Can you work these out from the model? Positions are in its coordinate system, mm. Face numbers are marked on the shaded views. A direction names the side the tool comes from. Round coordinates to 2 decimals unless told otherwise and drop trailing zeros. Loops run counter-clockwise (first coordinate to the right, second up) from the corner with the lowest first, then second, coordinate; pieces in that order, holes last.
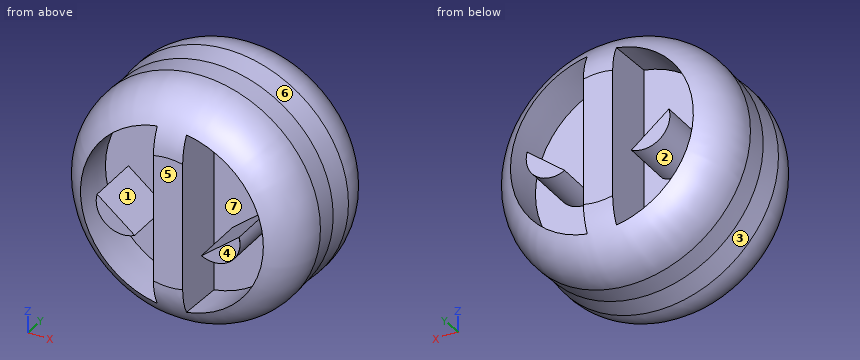
from build123d import *

# Parameters (mm, degrees)
F0_R         = 55.5262746105
F1_DEPTH     = 38.1
F1_TAPER     = -3
F2_DEPTH     = 38.1
F3_DEPTH     = 12.7
F4_DEPTH     = 38.1
F5_S5_R      = 12.3526687507
F5_T6_DEPTH  = 90
F5_S7_R      = 12.3526687507
F5_T8_DEPTH  = 90
F5_S13_R     = 12.3526687507
F5_T14_DEPTH = 90
F5_S15_R     = 12.3526687507
F5_T16_DEPTH = 90


# Not quite as in the source:
# - a fillet or chamfer that OpenCascade refuses, or shapes differently, is made with other operations: its cross-section is extruded or revolved along the edge and cut away or added
# - two fillets or chamfers of one size are made in one step


with BuildPart() as f1:
    # F0 (on Front) → F1 (new body, symmetric)
    with BuildSketch(Plane.XZ):
        Circle(F0_R)
        with BuildLine():
            ThreePointArc((6.861501839, 44.2620349836), (34.0113180152, 29.1451230097), (44.790712747, 0))
            ThreePointArc((44.790712747, 0), (34.0113180152, -29.1451230097), (6.861501839, -44.2620349836))
            Line((6.861501839, -44.2620349836), (6.861501839, -46.4376546443))
            Line((6.861501839, -46.4376546443), (-6.8615009077, -46.4376546443))
            Line((-6.8615009077, -46.4376546443), (-6.8615009077, -44.262035128))
            ThreePointArc((-6.8615009077, -44.262035128), (-44.790712747, 0), (-6.8615009077, 44.262035128))
            Line((-6.8615009077, 44.262035128), (-6.8615009077, 48.6431419849))
            Line((-6.8615009077, 48.6431419849), (6.861501839, 48.6431419849))
            Line((6.861501839, 48.6431419849), (6.861501839, 44.2620349836))
        make_face(mode=Mode.SUBTRACT)
        with BuildLine():
            ThreePointArc((-6.8615009077, 44.262035128), (4.712e-07, 44.790712747), (6.861501839, 44.2620349836))
            Line((6.861501839, 44.2620349836), (6.861501839, 48.6431419849))
            Line((6.861501839, 48.6431419849), (-6.8615009077, 48.6431419849))
            Line((-6.8615009077, 48.6431419849), (-6.8615009077, 44.262035128))
        make_face()
        with BuildLine():
            Line((6.861501839, -46.4376546443), (6.861501839, -44.2620349836))
            ThreePointArc((6.861501839, -44.2620349836), (4.712e-07, -44.790712747), (-6.8615009077, -44.262035128))
            Line((-6.8615009077, -44.262035128), (-6.8615009077, -46.4376546443))
            Line((-6.8615009077, -46.4376546443), (6.861501839, -46.4376546443))
        make_face()
    extrude(amount=F1_DEPTH, both=True, taper=F1_TAPER)

    # F0 (on Front) → F2 (join, symmetric)
    with BuildSketch(Plane.XZ):
        with BuildLine():
            Line((6.861501839, -44.2620349836), (6.861501839, 44.2620349836))
            ThreePointArc((6.861501839, 44.2620349836), (4.712e-07, 44.790712747), (-6.8615009077, 44.262035128))
            Line((-6.8615009077, 44.262035128), (-6.8615009077, -44.262035128))
            ThreePointArc((-6.8615009077, -44.262035128), (4.712e-07, -44.790712747), (6.861501839, -44.2620349836))
        make_face()
    extrude(amount=F2_DEPTH, both=True)

    # F0 (on Front) → F3 (join, symmetric)
    with BuildSketch(Plane.XZ):
        with BuildLine():
            Line((-6.8615009077, -44.262035128), (-6.8615009077, 44.262035128))
            ThreePointArc((-6.8615009077, 44.262035128), (-44.790712747, 0), (-6.8615009077, -44.262035128))
        make_face()
        with BuildLine():
            ThreePointArc((-15.6834311783, -10.942174576), (-29.1647493256, -9.6196886086), (-33.3272889256, 3.270934813))
            Line((-33.3272889256, 3.270934813), (-15.6834311783, -10.942174576))
        make_face(mode=Mode.SUBTRACT)
        with BuildLine():
            ThreePointArc((6.861501839, -44.2620349836), (34.0113180152, -29.1451230097), (44.790712747, 0))
            ThreePointArc((44.790712747, 0), (34.0113180152, 29.1451230097), (6.861501839, 44.2620349836))
            Line((6.861501839, 44.2620349836), (6.861501839, -44.2620349836))
        make_face()
        with BuildLine():
            Line((15.6834311783, -10.942174576), (33.3272889256, 3.270934813))
            ThreePointArc((33.3272889256, 3.270934813), (29.1647493256, -9.6196886086), (15.6834311783, -10.942174576))
        make_face(mode=Mode.SUBTRACT)
    extrude(amount=F3_DEPTH, both=True)

    # F0 (on Front) → F4 (join, symmetric)
    with BuildSketch(Plane.XZ):
        with BuildLine():
            Line((-15.6834311783, -10.942174576), (-33.3272889256, 3.270934813))
            ThreePointArc((-33.3272889256, 3.270934813), (-29.1647493256, -9.6196886086), (-15.6834311783, -10.942174576))
        make_face()
        with BuildLine():
            ThreePointArc((15.6834311783, -10.942174576), (29.1647493256, -9.6196886086), (33.3272889256, 3.270934813))
            Line((33.3272889256, 3.270934813), (15.6834311783, -10.942174576))
        make_face()
    extrude(amount=F4_DEPTH, both=True)

    # F5: fillet of radius 25.4 on 2 edges, made by hand


with BuildPart() as f5_tool2:
    # F5_s3 → F5_t4 (revolve)
    with BuildSketch(Plane.XY):
        with BuildLine():
            ThreePointArc((30.7569958191, 38.1), (49.1815048428, 30.1842062226), (56.1221860018, 11.3706667114))
            Line((56.1221860018, 11.3706667114), (57.5230110012, 38.1))
            Line((57.5230110012, 38.1), (30.7569958191, 38.1))
        make_face()
    revolve(axis=Axis((0, 38.1, 0), (0, -1, 0)))

    # F5_s5 → F5_t6 (cut, symmetric)
    with BuildSketch(Plane.XZ.offset(-16.4)):
        with Locations((-21.415554765, 0)):
            Circle(F5_S5_R)
    extrude(amount=F5_T6_DEPTH, both=True, mode=Mode.SUBTRACT)

    # F5_s7 → F5_t8 (cut, symmetric)
    with BuildSketch(Plane.XZ.offset(-16.4)):
        with Locations((21.415554765, 0)):
            Circle(F5_S7_R)
    extrude(amount=F5_T8_DEPTH, both=True, mode=Mode.SUBTRACT)


with BuildPart() as f1_1:
    add(f1.part)

    # F5_t1: cut F5_tool2
    add(f5_tool2.part, mode=Mode.SUBTRACT)


with BuildPart() as f5_tool10:
    # F5_s11 → F5_t12 (revolve)
    with BuildSketch(Plane.XY):
        with BuildLine():
            ThreePointArc((56.1221860018, -11.3706667114), (49.1815048428, -30.1842062226), (30.7569958191, -38.1))
            Line((30.7569958191, -38.1), (57.5230110012, -38.1))
            Line((57.5230110012, -38.1), (56.1221860018, -11.3706667114))
        make_face()
    revolve(axis=Axis((0, -38.1, 0), (0, 1, 0)))

    # F5_s13 → F5_t14 (cut, symmetric)
    with BuildSketch(Plane.XZ.offset(16.4)):
        with Locations((21.415554765, 0)):
            Circle(F5_S13_R)
    extrude(amount=F5_T14_DEPTH, both=True, mode=Mode.SUBTRACT)

    # F5_s15 → F5_t16 (cut, symmetric)
    with BuildSketch(Plane.XZ.offset(16.4)):
        with Locations((-21.415554765, 0)):
            Circle(F5_S15_R)
    extrude(amount=F5_T16_DEPTH, both=True, mode=Mode.SUBTRACT)


with BuildPart() as f1_2:
    add(f1_1.part)

    # F5_t9: cut F5_tool10
    add(f5_tool10.part, mode=Mode.SUBTRACT)


solid = f1_2.part
(1) If we section it at B-B, the plane y = 29: List the corners of the cut face in (x, z) for me.
Worked answers:
outline: circle Ø100.47 at (0, 0); (-33.33, 3.27) arc R12.35 ccw to (-15.68, -10.94) - close; (15.68, -10.94) arc R12.35 ccw to (33.33, 3.27) - close; hole (-6.86, -42.72) - (-6.86, 42.72) arc R43.27 ccw to start; hole (6.86, -42.72) arc R43.27 ccw to (6.86, 42.72) - close
(2) Will these pins go through, and if not, where does the flat tip stop? P1, Ø4, axis at x = 24.5, y = -23, coming from the -Z side; P2, Ø10, axis at y = -18, z = -6, coming from the +X side; P3, Ø6, axis at x = -35, y = -21.5, coming from the -Z side.
Worked answers:
P1: stops at z = -49.43
P2: stops at x = 56.05
P3: stops at z = -44.55
(3) If we mould it in two halves opening along X, with no side actions, what happens to the marked faces 5, 6 and 7? For each: released by +X, released by -X, zero draft, split by the parting line, or undercut.
Worked answers:
face 5: zero draft
face 6: split by the parting line
face 7: undercut
(4) If we section it at C-C, the plane y = 6.5: List the corners of the cut face in (x, z) for me.
Worked answers:
outline: circle Ø111.73 at (0, 0)
(5) If we section it at A-A, the plane y = -25.5: List the corners of the cut face in (x, z) for me, then the cut area to 3 significant figures.
Worked answers:
outline: circle Ø105.39 at (0, 0); (-33.33, 3.27) arc R12.35 ccw to (-15.68, -10.94) - close; (15.68, -10.94) arc R12.35 ccw to (33.33, 3.27) - close; hole (-6.86, -42.91) - (-6.86, 42.91) arc R43.45 ccw to start; hole (6.86, -42.91) arc R43.45 ccw to (6.86, 42.91) - close
area: 4,220 mm2
(6) For the marked faces 1, 2, 3 and 4, which set-ups out of +Z, -Z, +X, -X, +Y, -Y let a thin tool reach every point of the face, with its end or its side?
Worked answers:
face 1: -Y
face 2: +Y
face 3: none
face 4: +Z, -Z, +X, -X, -Y
(7) If I drill on line 1 (X direction, y = 30, z = -16); line 2 (X direction, y = 34, z = -14); line 3 (Z direction, x = 21, y = -32), over which ranges is the centre line in solid material (lowest first)?
Worked answers:
line 1: x = -46.69 to -40.15, -6.86 to 6.86, 40.15 to 46.69
line 2: x = -42.34 to -40.67, -6.86 to 6.86, 40.67 to 42.34
line 3: z = -42.35 to -37.65, -12.35 to -6.66, 37.65 to 42.35
